Verification items for the finished model (mm, model axes). Face numbers are marked on the shaded views. A direction names the side the tool comes from. Give positions to 0.01 mm unless a question says otherwise; leave off trailing zeros. Order: outer loops, then holes, each group sorted by start corner. A loop starts at its lowest first (then second) coordinate and runs counter-clockwise, first axis right, second up.
from build123d import *

# Parameters (mm, degrees)
SKETCH_1_W             = 630
SKETCH_1_H             = 42
EXTRUDE_1_DEPTH        = 9.5
SKETCH_2_R             = 4
CUT_EXTRUDE_1_DEPTH    = 4.5
SKETCH_3_R             = 2.25
CUT_EXTRUDE_2_DEPTH    = 632.418244906
SKETCH_16_W            = 5.144238896
SKETCH_16_H            = 2
SKETCH_16_W_2          = 7.201213672
CUT_EXTRUDE_6_DEPTH    = 632.469912189
SKETCH_6_W             = 56
SKETCH_6_H             = 60
EXTRUDE_2_DEPTH        = 12
HOLE_WIZARD_M4_1_D     = 3.3
HOLE_WIZARD_M4_1_DEPTH = 7
HOLE_WIZARD_M4_1_TIP   = 0.991420021
SKETCH_9_W             = 5
SKETCH_9_H             = 60
CUT_EXTRUDE_3_DEPTH    = 2
SKETCH_10_W            = 46
SKETCH_10_H            = 20
CUT_EXTRUDE_4_DEPTH    = 1
SKETCH_11_W            = 1.5
SKETCH_11_H            = 60
CUT_EXTRUDE_5_DEPTH    = 1
HOLE_WIZARD_M4_2_D     = 3.3


with BuildPart() as part:
    # 스케치1 → 보스-돌출1 (new body)
    with BuildSketch(Plane(origin=(0, 0, 0), x_dir=(1, 0, 0), z_dir=(0, 1, 0))):
        with Locations((315, 21)):
            Rectangle(SKETCH_1_W, SKETCH_1_H)
    extrude(amount=EXTRUDE_1_DEPTH)

    # 스케치2 → 컷-돌출1 (cut)
    with BuildSketch(Plane(origin=(0, 9.5, 0), x_dir=(1, 0, 0), z_dir=(0, 1, 0))):
        with Locations(Location((35, 32.5, 0), (0, 0, 270))):
            Circle(SKETCH_2_R)
        with Locations(Location((35, 9.5, 0), (0, 0, 270))):
            Circle(SKETCH_2_R)
        with Locations(Location((75, 32.5, 0), (0, 0, 270))):
            Circle(SKETCH_2_R)
        with Locations(Location((75, 9.5, 0), (0, 0, 270))):
            Circle(SKETCH_2_R)
        with Locations(Location((115, 32.5, 0), (0, 0, 270))):
            Circle(SKETCH_2_R)
        with Locations(Location((115, 9.5, 0), (0, 0, 270))):
            Circle(SKETCH_2_R)
        with Locations(Location((155, 32.5, 0), (0, 0, 270))):
            Circle(SKETCH_2_R)
        with Locations(Location((155, 9.5, 0), (0, 0, 270))):
            Circle(SKETCH_2_R)
        with Locations(Location((195, 32.5, 0), (0, 0, 270))):
            Circle(SKETCH_2_R)
        with Locations(Location((195, 9.5, 0), (0, 0, 270))):
            Circle(SKETCH_2_R)
        with Locations(Location((235, 32.5, 0), (0, 0, 270))):
            Circle(SKETCH_2_R)
        with Locations(Location((235, 9.5, 0), (0, 0, 270))):
            Circle(SKETCH_2_R)
        with Locations(Location((275, 32.5, 0), (0, 0, 270))):
            Circle(SKETCH_2_R)
        with Locations(Location((275, 9.5, 0), (0, 0, 270))):
            Circle(SKETCH_2_R)
        with Locations(Location((315, 32.5, 0), (0, 0, 270))):
            Circle(SKETCH_2_R)
        with Locations(Location((315, 9.5, 0), (0, 0, 270))):
            Circle(SKETCH_2_R)
        with Locations(Location((355, 32.5, 0), (0, 0, 270))):
            Circle(SKETCH_2_R)
        with Locations(Location((355, 9.5, 0), (0, 0, 270))):
            Circle(SKETCH_2_R)
        with Locations(Location((395, 32.5, 0), (0, 0, 270))):
            Circle(SKETCH_2_R)
        with Locations(Location((395, 9.5, 0), (0, 0, 270))):
            Circle(SKETCH_2_R)
        with Locations(Location((435, 32.5, 0), (0, 0, 270))):
            Circle(SKETCH_2_R)
        with Locations(Location((435, 9.5, 0), (0, 0, 270))):
            Circle(SKETCH_2_R)
        with Locations(Location((475, 32.5, 0), (0, 0, 270))):
            Circle(SKETCH_2_R)
        with Locations(Location((475, 9.5, 0), (0, 0, 270))):
            Circle(SKETCH_2_R)
        with Locations(Location((515, 32.5, 0), (0, 0, 270))):
            Circle(SKETCH_2_R)
        with Locations(Location((515, 9.5, 0), (0, 0, 270))):
            Circle(SKETCH_2_R)
        with Locations(Location((555, 32.5, 0), (0, 0, 270))):
            Circle(SKETCH_2_R)
        with Locations(Location((555, 9.5, 0), (0, 0, 270))):
            Circle(SKETCH_2_R)
        with Locations(Location((595, 32.5, 0), (0, 0, 270))):
            Circle(SKETCH_2_R)
        with Locations(Location((595, 9.5, 0), (0, 0, 270))):
            Circle(SKETCH_2_R)
    extrude(amount=-CUT_EXTRUDE_1_DEPTH, mode=Mode.SUBTRACT)

    # 스케치3 → 컷-돌출2 (cut, through all)
    with BuildSketch(Plane(origin=(0, 5, 0), x_dir=(1, 0, 0), z_dir=(0, 1, 0))):
        with Locations(Location((35, 32.5, 0), (0, 0, 270))):
            Circle(SKETCH_3_R)
        with Locations(Location((35, 9.5, 0), (0, 0, 270))):
            Circle(SKETCH_3_R)
        with Locations(Location((75, 32.5, 0), (0, 0, 270))):
            Circle(SKETCH_3_R)
        with Locations(Location((75, 9.5, 0), (0, 0, 270))):
            Circle(SKETCH_3_R)
        with Locations(Location((115, 32.5, 0), (0, 0, 270))):
            Circle(SKETCH_3_R)
        with Locations(Location((115, 9.5, 0), (0, 0, 270))):
            Circle(SKETCH_3_R)
        with Locations(Location((155, 32.5, 0), (0, 0, 270))):
            Circle(SKETCH_3_R)
        with Locations(Location((155, 9.5, 0), (0, 0, 270))):
            Circle(SKETCH_3_R)
        with Locations(Location((195, 32.5, 0), (0, 0, 270))):
            Circle(SKETCH_3_R)
        with Locations(Location((195, 9.5, 0), (0, 0, 270))):
            Circle(SKETCH_3_R)
        with Locations(Location((235, 32.5, 0), (0, 0, 270))):
            Circle(SKETCH_3_R)
        with Locations(Location((235, 9.5, 0), (0, 0, 270))):
            Circle(SKETCH_3_R)
        with Locations(Location((275, 32.5, 0), (0, 0, 270))):
            Circle(SKETCH_3_R)
        with Locations(Location((275, 9.5, 0), (0, 0, 270))):
            Circle(SKETCH_3_R)
        with Locations(Location((315, 32.5, 0), (0, 0, 270))):
            Circle(SKETCH_3_R)
        with Locations(Location((315, 9.5, 0), (0, 0, 270))):
            Circle(SKETCH_3_R)
        with Locations(Location((355, 32.5, 0), (0, 0, 270))):
            Circle(SKETCH_3_R)
        with Locations(Location((355, 9.5, 0), (0, 0, 270))):
            Circle(SKETCH_3_R)
        with Locations(Location((395, 32.5, 0), (0, 0, 270))):
            Circle(SKETCH_3_R)
        with Locations(Location((395, 9.5, 0), (0, 0, 270))):
            Circle(SKETCH_3_R)
        with Locations(Location((435, 32.5, 0), (0, 0, 270))):
            Circle(SKETCH_3_R)
        with Locations(Location((435, 9.5, 0), (0, 0, 270))):
            Circle(SKETCH_3_R)
        with Locations(Location((475, 32.5, 0), (0, 0, 270))):
            Circle(SKETCH_3_R)
        with Locations(Location((475, 9.5, 0), (0, 0, 270))):
            Circle(SKETCH_3_R)
        with Locations(Location((515, 32.5, 0), (0, 0, 270))):
            Circle(SKETCH_3_R)
        with Locations(Location((515, 9.5, 0), (0, 0, 270))):
            Circle(SKETCH_3_R)
        with Locations(Location((555, 32.5, 0), (0, 0, 270))):
            Circle(SKETCH_3_R)
        with Locations(Location((555, 9.5, 0), (0, 0, 270))):
            Circle(SKETCH_3_R)
        with Locations(Location((595, 32.5, 0), (0, 0, 270))):
            Circle(SKETCH_3_R)
        with Locations(Location((595, 9.5, 0), (0, 0, 270))):
            Circle(SKETCH_3_R)
    extrude(amount=-CUT_EXTRUDE_2_DEPTH, mode=Mode.SUBTRACT)

    # 스케치16 → 컷-돌출6 (cut, through all)
    with BuildSketch(Plane(origin=(630, 0, 0), x_dir=(0, 0, -1), z_dir=(1, 0, 0))):
        with Locations((-0.572119448, 5)):
            Rectangle(SKETCH_16_W, SKETCH_16_H)
        with Locations((43.600606836, 5)):
            Rectangle(SKETCH_16_W_2, SKETCH_16_H)
    extrude(amount=-CUT_EXTRUDE_6_DEPTH, mode=Mode.SUBTRACT)

    # 스케치6 → 보스-돌출2 (add)
    with BuildSketch(Plane(origin=(0, 4, 0), x_dir=(-1, 0, 0), z_dir=(0, -1, 0))):
        with Locations((-518, 21)):
            Rectangle(SKETCH_6_W, SKETCH_6_H)
    extrude(amount=-EXTRUDE_2_DEPTH)

    # M4 나사 구멍1
    with Locations(Plane(origin=(0, 16, 0), x_dir=(1, 0, 0), z_dir=(0, 1, 0))):
        with Locations((508, 43.5), (528, 43.5), (508, -1.5), (528, -1.5)):
            Hole(HOLE_WIZARD_M4_1_D / 2, depth=HOLE_WIZARD_M4_1_DEPTH)
            with Locations((0, 0, -(HOLE_WIZARD_M4_1_DEPTH + HOLE_WIZARD_M4_1_TIP / 2))):  # 118° drill point
                Cone(0, HOLE_WIZARD_M4_1_D / 2, HOLE_WIZARD_M4_1_TIP, mode=Mode.SUBTRACT)

    # 스케치9 → 컷-돌출3 (cut)
    with BuildSketch(Plane(origin=(0, 16, 0), x_dir=(1, 0, 0), z_dir=(0, 1, 0))):
        with Locations((492.5, 21)):
            Rectangle(SKETCH_9_W, SKETCH_9_H)
        with Locations((543.5, 21)):
            Rectangle(SKETCH_9_W, SKETCH_9_H)
    extrude(amount=-CUT_EXTRUDE_3_DEPTH, mode=Mode.SUBTRACT)

    # 스케치10 → 컷-돌출4 (cut)
    with BuildSketch(Plane(origin=(0, 16, 0), x_dir=(1, 0, 0), z_dir=(0, 1, 0))):
        with Locations((518, 21)):
            Rectangle(SKETCH_10_W, SKETCH_10_H)
    extrude(amount=-CUT_EXTRUDE_4_DEPTH, mode=Mode.SUBTRACT)

    # 스케치11 → 컷-돌출5 (cut)
    with BuildSketch(Plane(origin=(0, 14, 0), x_dir=(1, 0, 0), z_dir=(0, 1, 0))):
        with Locations((545.25, 21)):
            Rectangle(SKETCH_11_W, SKETCH_11_H)
        with Locations((490.75, 21)):
            Rectangle(SKETCH_11_W, SKETCH_11_H)
    extrude(amount=-CUT_EXTRUDE_5_DEPTH, mode=Mode.SUBTRACT)

    # M4 나사 구멍2 (through all)
    with Locations(Plane.XY.offset(9)):
        with Locations((518, 12.75)):
            Hole(HOLE_WIZARD_M4_2_D / 2)


solid = part.part
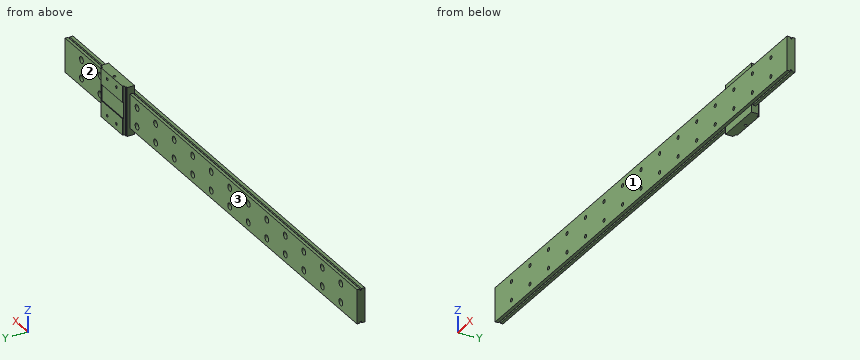
(1) Go/stop test with flat-tipped pins: pin 1 (2.5 mm diameter, centred on x = 528.5, z = 2.5, fed in from -Y); pin 2 (2 mm diameter, centred on x = 283.5, z = -1, fed in from +Y); pin 3 (3 mm diameter, centred on x = 282, y = 5.5, fed in from +Z). Record where each tip stops, or that it passes through.
Solved:
pin 1: stops at y = 4
pin 2: stops at y = 9.5
pin 3: stops at z = 0
(2) Section check A-A, the plane z = -21. Enter the section's corners in (x, y).
Solved:
outline: (0, 0) - (630, 0) - (630, 9.5) - (546, 9.5) - (546, 13) - (544.5, 13) - (544.5, 14) - (541, 14) - (541, 15) - (495, 15) - (495, 14) - (491.5, 14) - (491.5, 13) - (490, 13) - (490, 9.5) - (0, 9.5) - close; hole circle Ø3.3 at (518, 12.75)
(3) Scan lines: line 1 (Z direction, x = 435, y = 6.25); line 2 (Z direction, x = 155, y = 2.2); line 3 (Y direction, x = 82.5, z = -41). Record each from-to range of solid material in increasing order.
Solved:
line 1: z = -42 to -36.5, -28.5 to -13.5, -5.5 to 0
line 2: z = -42 to -34.75, -30.25 to -11.75, -7.25 to 0
line 3: y = 0 to 4, 6 to 9.5
(4) Set-up check for the marked faces 1, 2 and 3: record each of +Z, -Z, +X, -X, +Y, -Y from which the full face is reachable in a straight line by a thin tool's end or side.
Solved:
face 1: +Z, -Z, +X, -X, -Y
face 2: +Z, -Z, +X, +Y
face 3: +Z, -Z, -X, +Y
(5) Section check B-B, the plane x = 584. Enter the section's corners in (y, z), then the cut area to 3 significant figures.
Solved:
outline: (0, -42) - (4, -42) - (4, -40) - (6, -40) - (6, -42) - (9.5, -42) - (9.5, 0) - (6, 0) - (6, -2) - (4, -2) - (4, 0) - (0, 0) - close
area: 391 mm2
